from build123d import *

# Parameters (mm, degrees)
SKETCH1_R           = 175
BOSS_EXTRUDE1_DEPTH = 6
SKETCH2_W           = 80
SKETCH2_H           = 20
SKETCH2_W_2         = 60
SKETCH2_H_2         = 60
CUT_EXTRUDE1_DEPTH  = 248.560093715
SKETCH3_W           = 10
SKETCH3_H           = 6
CUT_EXTRUDE2_DEPTH  = 248.560093715
SKETCH4_R           = 1.5
CUT_EXTRUDE3_DEPTH  = 248.560093715
SKETCH5_R           = 1.5
CUT_EXTRUDE4_DEPTH  = 248.560093715
SKETCH6_R           = 8.5
CUT_EXTRUDE5_DEPTH  = 248.560093715
CAVITY1_OUTLINE_R   = 1.5
CAVITY1_DEPTH       = 6
SKETCH7_W           = 35
SKETCH7_H           = 160
CUT_EXTRUDE6_DEPTH  = 248.560093715
SKETCH8_R           = 1.5
CUT_EXTRUDE7_DEPTH  = 10


# Read off the part's stored shape, not the designer's step: Cavity1
with BuildPart() as part:
    # Sketch1 → Boss-Extrude1 (new body)
    with BuildSketch(Plane.XY):
        Circle(SKETCH1_R)
    extrude(amount=BOSS_EXTRUDE1_DEPTH)

    # Sketch2 → Cut-Extrude1 (cut, through all)
    with BuildSketch(Plane(origin=(0, 0, 0), x_dir=(-1, 0, 0), z_dir=(0, 0, -1))):
        with Locations((0, 130)):
            Rectangle(SKETCH2_W, SKETCH2_H)
        with Locations((0, -130)):
            Rectangle(SKETCH2_W, SKETCH2_H)
        with Locations((-100, 0)):
            Rectangle(SKETCH2_W_2, SKETCH2_H_2)
    extrude(amount=-CUT_EXTRUDE1_DEPTH, mode=Mode.SUBTRACT)

    # Sketch3 → Cut-Extrude2 (cut, through all)
    with BuildSketch(Plane.XY.offset(6)):
        with Locations((75, 33)):
            Rectangle(SKETCH3_W, SKETCH3_H)
        with Locations((125, 33)):
            Rectangle(SKETCH3_W, SKETCH3_H)
        with Locations((75, -33)):
            Rectangle(SKETCH3_W, SKETCH3_H)
        with Locations((125, -33)):
            Rectangle(SKETCH3_W, SKETCH3_H)
    extrude(amount=-CUT_EXTRUDE2_DEPTH, mode=Mode.SUBTRACT)

    # Sketch4 → Cut-Extrude3 (cut, through all)
    with BuildSketch(Plane.XY.offset(6)):
        with Locations((-30, -157)):
            Circle(SKETCH4_R)
        with Locations((45, -157)):
            Circle(SKETCH4_R)
        with Locations(Location((-30, 157, 0), (0, 0, 180))):
            Circle(SKETCH4_R)
        with Locations(Location((45, 157, 0), (0, 0, 180))):
            Circle(SKETCH4_R)
        with Locations(Location((45, -93.75, 0), (0, 0, 180))):
            Circle(SKETCH4_R)
        with Locations(Location((-30, -93.75, 0), (0, 0, 180))):
            Circle(SKETCH4_R)
        with Locations((45, 93.75)):
            Circle(SKETCH4_R)
        with Locations((-30, 93.75)):
            Circle(SKETCH4_R)
    extrude(amount=-CUT_EXTRUDE3_DEPTH, mode=Mode.SUBTRACT)

    # Sketch5 → Cut-Extrude4 (cut, through all)
    with BuildSketch(Plane.XY.offset(6)):
        with Locations((89.5, 88.5)):
            Circle(SKETCH5_R)
        with Locations((130.5, 88.5)):
            Circle(SKETCH5_R)
        with Locations((130.5, 47.5)):
            Circle(SKETCH5_R)
        with Locations((89.5, 47.5)):
            Circle(SKETCH5_R)
        with Locations(Location((89.5, -88.5, 0), (0, 0, 180))):
            Circle(SKETCH5_R)
        with Locations(Location((130.5, -88.5, 0), (0, 0, 180))):
            Circle(SKETCH5_R)
        with Locations(Location((130.5, -47.5, 0), (0, 0, 180))):
            Circle(SKETCH5_R)
        with Locations(Location((89.5, -47.5, 0), (0, 0, 180))):
            Circle(SKETCH5_R)
    extrude(amount=-CUT_EXTRUDE4_DEPTH, mode=Mode.SUBTRACT)

    # Sketch6 → Cut-Extrude5 (cut, through all)
    with BuildSketch(Plane.XY.offset(6)):
        with Locations((155, 12.5)):
            Circle(SKETCH6_R)
        with Locations((155, -12.5)):
            Circle(SKETCH6_R)
    extrude(amount=-CUT_EXTRUDE5_DEPTH, mode=Mode.SUBTRACT)

    # Cavity1 outline → Cavity1 (cut)
    with BuildSketch(Plane.XY):
        with Locations((72.337603572, -125.375)):
            Circle(CAVITY1_OUTLINE_R)
        with Locations((72.337603572, 125.375)):
            Circle(CAVITY1_OUTLINE_R)
    extrude(amount=CAVITY1_DEPTH, mode=Mode.SUBTRACT)

    # Sketch7 → Cut-Extrude6 (cut, through all)
    with BuildSketch(Plane.XY.offset(6)):
        with Locations((42.5, 0)):
            Rectangle(SKETCH7_W, SKETCH7_H)
    extrude(amount=-CUT_EXTRUDE6_DEPTH, mode=Mode.SUBTRACT)

    # Sketch8 → Cut-Extrude7 (cut)
    with BuildSketch(Plane.XY.offset(6)):
        with Locations((15, 37.5)):
            Circle(SKETCH8_R)
        with Locations((-45, -37.5)):
            Circle(SKETCH8_R)
        Polygon((-15, 32.5), (20, 32.5), (20, -32.5), (20, -42.5), (-15, -42.5), (-15, -32.5), (-50, -32.5), (-50, 42.5), (-15, 42.5), align=None)
    extrude(amount=-CUT_EXTRUDE7_DEPTH, mode=Mode.SUBTRACT)


solid = part.part
The listing builds one solid part. Answer for the finished solid, in the listing's coordinates (mm). Give positions to 0.01 mm unless a question says otherwise; leave off trailing zeros. Write each loop counter-clockwise with the first axis right and the second up, starting at its lowest first coordinate (ties: lowest second). Pieces come first, ordered by that corner, then holes. Notation, with made-up numbers: (58.5, 3.25) -> (90.5, 3.25) arc R15 ccw to (90.5, 18.25) -> close; hole circle Ø6 at (66, 82). An arc over 180 degrees is marked (long way). Use a Markdown table: item, result.
(1) Section B-B, the plane y = 54 is taken. Determine the outline of the cut face in (x, z), then the cut area to 3 significant figures.
Return value:
| item | result |
|---|---|
| outline | (-166.46, 0) -> (25, 0) -> (25, 6) -> (-166.46, 6) -> close; (60, 0) -> (166.46, 0) -> (166.46, 6) -> (60, 6) -> close |
| area | 1,790 mm2 |
(2) Section D-D, the plane z = 2.75 is taken. Give the number of separate pieces and of enclosed holes in the cut face, then the cut area to 3 significant figures.
Return value:
| item | result |
|---|---|
| separate pieces | 1 |
| enclosed holes | 27 |
| area | 77,700 mm2 |
(3) Determine the mould class of faces 1 (the cylindrical face through (-128.982, 118.273, 2.958)), 2 (the cylindrical face through (163.11, -9.95, 3.04)), 3 (the cylindrical face through (162.85, 9.24, 3.04)), 4 (the flat face through (-2, 41, 0)) for opening direction Y: released by +Y, released by -Y, zero draft, split by the parting line, or undercut.
Return value:
| item | result |
|---|---|
| face 1 | split by the parting line |
| face 2 | undercut |
| face 3 | undercut |
| face 4 | zero draft |
(4) Section A-A, the plane y = 0 is taken. Determine the outline of the cut face in (x, z).
Return value:
| item | result |
|---|---|
| outline | (-175, 0) -> (-50, 0) -> (-50, 6) -> (-175, 6) -> close; (20, 0) -> (25, 0) -> (25, 6) -> (20, 6) -> close; (60, 0) -> (70, 0) -> (70, 6) -> (60, 6) -> close; (130, 0) -> (175, 0) -> (175, 6) -> (130, 6) -> close |
(5) Find the intervals of material crossed by probe 1 along X at (y, z) = (37, 3.35); probe 2 along Y at (x, z) = (89.5, 3.6); probe 3 along Y at (x, z) = (45, 3), in increasing order. Write a range as from..to.
Return value:
| item | result |
|---|---|
| probe 1 | -171.04..-50, -15..13.59, 16.41..25, 60..171.04 |
| probe 2 | -150.38..-90, -87..-49, -46..-30, 30..46, 49..87, 90..150.38 |
| probe 3 | -169.12..-158.5, -155.5..-95.25, -92.25..-80, 80..92.25, 95.25..155.5, 158.5..169.12 |
(6) Section C-C, the plane x = 155 is taken. Determine the outline of the cut face in (y, z), then the cut area to 3 significant figures.
Return value:
| item | result |
|---|---|
| outline | (-81.24, 0) -> (-21, 0) -> (-21, 6) -> (-81.24, 6) -> close; (-4, 0) -> (4, 0) -> (4, 6) -> (-4, 6) -> close; (21, 0) -> (81.24, 0) -> (81.24, 6) -> (21, 6) -> close |
| area | 771 mm2 |
(7) Flat-ended cylindrical pins translate along their axes: P1, Ø1.8, axis at y = -131.5, z = 3.5, coming from the -X side; P2, Ø3, axis at y = -138, z = 2, coming from the +X side; P3, Ø3, axis at x = -126, z = 1, coming from the -Y side. Find the tip coordinate at first contact, or state that the pin passes through.
Return value:
| item | result |
|---|---|
| P1 | x = -116.48 |
| P2 | x = 109.51 |
| P3 | y = -122.98 |
